from build123d import *

# Parameters (mm, degrees)
BOSS_EXTRUDE1_DEPTH         = 400.05
F_6_32_TAPPED_HOLE1_D       = 2.7051
F_6_CLEARANCE_HOLE1_D       = 3.7973
F_1_4_CLEARANCE_HOLE1_D     = 6.7564
F_1_4_CLEARANCE_HOLE1_DEPTH = 3.175
MIRROR3_COPY_1_D            = 6.7564
MIRROR3_COPY_1_DEPTH        = 3.175


with BuildPart() as part:
    # Sketch1 → Boss-Extrude1 (new, symmetric)
    with BuildSketch(Plane.XY):
        Polygon((-22.225, -15.875), (25.4, -15.875), (25.4, -19.05), (-25.4, -19.05), (-25.4, 19.05), (25.4, 19.05), (25.4, 15.875), (-22.225, 15.875), align=None)
    extrude(amount=BOSS_EXTRUDE1_DEPTH, both=True)

    # #6-32 Tapped Hole1 (through all)
    with Locations(Plane(origin=(0, 19.05, 0), x_dir=(1, 0, 0), z_dir=(0, 1, 0))):
        with Locations((15.875, -12.7)):
            f_6_32_tapped_hole1 = Hole(F_6_32_TAPPED_HOLE1_D / 2)

    # #6 Clearance Hole1 (through all)
    with Locations(Plane(origin=(0, 19.05, 0), x_dir=(1, 0, 0), z_dir=(0, 1, 0))):
        with Locations((20.32, -57.15)):
            f_6_clearance_hole1 = Hole(F_6_CLEARANCE_HOLE1_D / 2)

    # 1/4 Clearance Hole1
    with Locations(Plane(origin=(0, -19.05, 0), x_dir=(-1, 0, 0), z_dir=(0, -1, 0))):
        with Locations((-12.7, -374.65)):
            f_1_4_clearance_hole1 = Hole(F_1_4_CLEARANCE_HOLE1_D / 2, depth=F_1_4_CLEARANCE_HOLE1_DEPTH)

    # Mirror2: 1/4 Clearance Hole1 across plane
    add(f_1_4_clearance_hole1.mirror(Plane.ZX), mode=Mode.SUBTRACT)

    # Mirror3: 1/4 Clearance Hole1 across plane
    add(f_1_4_clearance_hole1.mirror(Plane.XY), mode=Mode.SUBTRACT)

    # Mirror3 copy 1
    with Locations(Plane(origin=(0, 19.05, 0), x_dir=(-1, 0, 0), z_dir=(0, 1, 0))):
        with Locations((-12.7, -374.65)):
            Hole(MIRROR3_COPY_1_D / 2, depth=MIRROR3_COPY_1_DEPTH)

    # Mirror4: #6-32 Tapped Hole1, #6 Clearance Hole1 across plane
    add(f_6_32_tapped_hole1.mirror(Plane.XY), mode=Mode.SUBTRACT)
    add(f_6_clearance_hole1.mirror(Plane.XY), mode=Mode.SUBTRACT)


solid = part.part
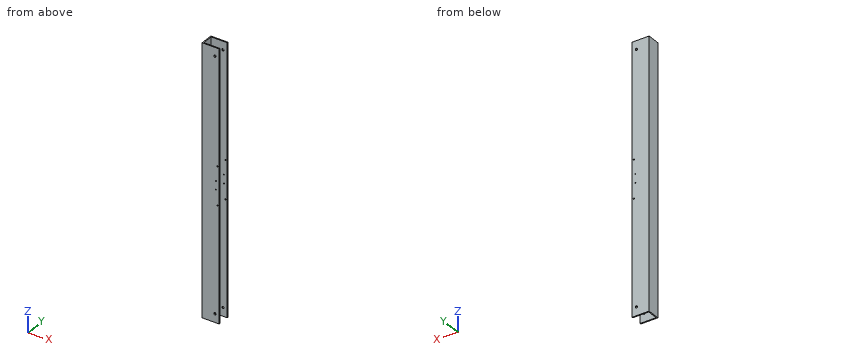
Model file for the job. Use its own axes, mm. Coordinates: 2 decimals unless noted, no trailing zeros. Write each loop counter-clockwise with the first axis right and the second up, starting at its lowest first coordinate (ties: lowest second). Pieces come first, ordered by that corner, then holes. Notation, with made-up numbers: (-1.5, 18) - (10.5, 18) arc R28 cw to (10.5, 56) - close; hole circle Ø10 at (60.5, -26.5). An arc over 180 degrees is marked (long way). Write each question's results on one line, items separated by ' | '. Start each with the question number.
1) Probe line 1 along Z through (x, y) = (12, 17); line 2 along Y through (x, z) = (-7, -332.5) (3 decimals); line 3 along X through (y, z) = (-18, 57). List the from-to ranges inside material, lowest first. Write a range as from..to.
2) Cut at A-A (x = -14). Write the cut outline in (y, z) (3 decimals).
3) Cut at C-C (y = -3). Write the cut outline in (x, z) (3 decimals), then the cut area to 3 significant figures.
4) Cut at B-B (z = -121). Write the cut outline in (x, y) (3 decimals).
5) Flat gauge pin, fed straight in: P1, Ø12, axis at y = -9, z = 284.5, coming from the +X side (3 decimals). Where does the tip first touch, or does it go through?
Returned:
1) line 1: -400.05..-377.95, -371.35..371.35, 377.95..400.05 | line 2: -19.05..-15.875, 15.875..19.05 | line 3: -25.4..18.43, 22.21..25.4
2) outline: (-19.05, -400.05) - (-15.875, -400.05) - (-15.875, 400.05) - (-19.05, 400.05) - close; (15.875, -400.05) - (19.05, -400.05) - (19.05, 400.05) - (15.875, 400.05) - close
3) outline: (-25.4, -400.05) - (-22.225, -400.05) - (-22.225, 400.05) - (-25.4, 400.05) - close | area: 2,540 mm^2
4) outline: (-25.4, -19.05) - (25.4, -19.05) - (25.4, -15.875) - (-22.225, -15.875) - (-22.225, 15.875) - (25.4, 15.875) - (25.4, 19.05) - (-25.4, 19.05) - close
5) P1: x = -22.225
